from build123d import *

# Parameters (mm, degrees)
SKETCH1_R                = 7.9375
BOSS_EXTRUDE1_DEPTH      = 4.7625
H_0_266_DIAMETER_HOLE1_D = 6.7564


with BuildPart() as part:
    # Sketch1 → Boss-Extrude1 (new body)
    with BuildSketch(Plane.XY):
        with BuildLine():
            Line((-31.75, 0), (-50.274457233, 62.375531935))
            ThreePointArc((-50.274457233, 62.375531935), (-44.45, 76.989658396), (-28.881566614, 74.726723093))
            Line((-28.881566614, 74.726723093), (15.875, 27.49630657))
            Line((15.875, 27.49630657), (78.9111987, 12.409785423))
            Line((78.9111987, 12.409785423), (130.763159277, 0))
            Line((130.763159277, 0), (79.156023847, -12.351191158))
            Line((79.156023847, -12.351191158), (15.875, -27.49630657))
            Line((15.875, -27.49630657), (-28.881566614, -74.726723093))
            ThreePointArc((-28.881566614, -74.726723093), (-44.45, -76.989658396), (-50.274457233, -62.375531935))
            Line((-50.274457233, -62.375531935), (-31.75, 0))
        make_face()
        Circle(SKETCH1_R, mode=Mode.SUBTRACT)
        with BuildLine():
            Line((9.968214912, 24.497802386), (-25.925542767, 62.375531935))
            ThreePointArc((-25.925542767, 62.375531935), (-31.75, 54.99261314), (-41.056023847, 53.639944611))
            Line((-41.056023847, 53.639944611), (-26.199826659, 3.616173849))
            ThreePointArc((-26.199826659, 3.616173849), (-6.35, 10.998522628), (9.968214912, 24.497802386))
        make_face(mode=Mode.SUBTRACT)
        with BuildLine():
            Line((16.231611747, 20.881628537), (66.981566614, 8.735587325))
            ThreePointArc((66.981566614, 8.735587325), (63.5, 0), (66.981566614, -8.735587325))
            Line((66.981566614, -8.735587325), (16.231611747, -20.881628537))
            ThreePointArc((16.231611747, -20.881628537), (12.7, 0), (16.231611747, 20.881628537))
        make_face(mode=Mode.SUBTRACT)
        with BuildLine():
            Line((88.374457233, 3.615603833), (103.481579639, 0))
            Line((103.481579639, 0), (88.374457233, -3.615603833))
            ThreePointArc((88.374457233, -3.615603833), (88.9, 0), (88.374457233, 3.615603833))
        make_face(mode=Mode.SUBTRACT)
        with BuildLine():
            Line((9.968214912, -24.497802386), (-25.925542767, -62.375531935))
            ThreePointArc((-25.925542767, -62.375531935), (-31.75, -54.99261314), (-41.056023847, -53.639944611))
            Line((-41.056023847, -53.639944611), (-26.199826659, -3.616173849))
            ThreePointArc((-26.199826659, -3.616173849), (-6.35, -10.998522628), (9.968214912, -24.497802386))
        make_face(mode=Mode.SUBTRACT)
    extrude(amount=-BOSS_EXTRUDE1_DEPTH)

    # H (0.266) Diameter Hole1 (through all)
    with Locations(Plane.XY):
        with Locations((76.2, 0), (-38.1, 65.991135768), (-38.1, -65.991135768)):
            Hole(H_0_266_DIAMETER_HOLE1_D / 2)


solid = part.part
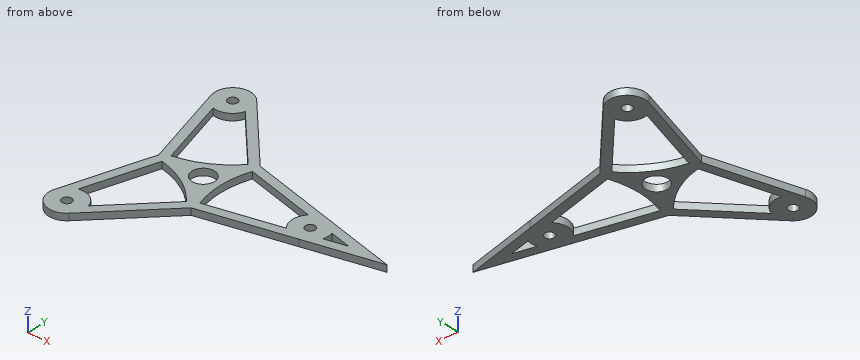
Here's how the part is built. I have some questions about the finished solid (model axes, mm). Give positions to 0.01 mm unless a question says otherwise; leave off trailing zeros. Loops run counter-clockwise (first coordinate to the right, second up) from the corner with the lowest first, then second, coordinate; pieces in that order, holes last. Notation, with made-up numbers: (68, 24) -> (101, 24) arc R24 ccw to (101, 52) -> close; hole circle Ø8 at (46.5, 2.5). An arc over 180 degrees is marked (long way). Answer as a JSON object with one key per item and string values. Group by question number.
Item 1: Imagine slicing it at A-A on x = -38.1. Write out the boundary of the cut face in (y, z), then the cut area to 3 significant figures.
Item 2: Will these pins go through, and if not, where does the flat tip stop? pin 1 (9 mm diameter, centred on x = -38.1, y = -65.99, fed in from +Z); pin 2 (1.5 mm diameter, centred on x = -3, z = -4, fed in from -Y).
Item 3: Imagine slicing it at C-C on y = -44. Write out the boundary of the cut face in (x, z).
Item 4: Imagine slicing it at D-D on z = -3.5. Give the number of separate pieces and of enclosed holes in the cut face, then the cut area to 3 significant figures.
Item 5: Imagine slicing it at B-B on x = 99.5. Write out the boundary of the cut face in (y, z).
Item 6: I need wall thicknesses on L1, parallel to Y at x = 9, z = -4.35; L2, parallel to Y at x = 0, z = -3.05; L3, parallel to Y at x = -2, z = -3.15. Which ranges of each line are inside material? Lowest first, please.
Answer list:
{
 "1": {"outline": "(-78.69, -4.76) -> (-69.37, -4.76) -> (-69.37, 0) -> (-78.69, 0) -> close; (-62.61, -4.76) -> (-53.29, -4.76) -> (-53.29, 0) -> (-62.61, 0) -> close; (-43.69, -4.76) -> (-21.38, -4.76) -> (-21.38, 0) -> (-43.69, 0) -> close; (21.38, -4.76) -> (43.69, -4.76) -> (43.69, 0) -> (21.38, 0) -> close; (53.29, -4.76) -> (62.61, -4.76) -> (62.61, 0) -> (53.29, 0) -> close; (69.37, -4.76) -> (78.69, -4.76) -> (78.69, 0) -> (69.37, 0) -> close", "area": "390 mm2"},
 "2": {"pin 1": "stops at z = 0", "pin 2": "stops at y = -48.21"},
 "3": {"outline": "(-44.82, -4.76) -> (-38.19, -4.76) -> (-38.19, 0) -> (-44.82, 0) -> close; (-8.51, -4.76) -> (0.24, -4.76) -> (0.24, 0) -> (-8.51, 0) -> close"},
 "4": {"separate pieces": "1", "enclosed holes": "8", "area": "4,830 mm2"},
 "5": {"outline": "(-7.48, -4.76) -> (-0.95, -4.76) -> (-0.95, 0) -> (-7.48, 0) -> close; (0.95, -4.76) -> (7.48, -4.76) -> (7.48, 0) -> (0.95, 0) -> close"},
 "6": {"L1": "y = -34.75 to -25.52, -23.4 to 23.4, 25.52 to 34.75", "L2": "y = -44.25 to -35.02, -15.19 to -7.94, 7.94 to 15.19, 35.02 to 44.25", "L3": "y = -46.36 to -37.13, -13.75 to -7.68, 7.68 to 13.75, 37.13 to 46.36"}
}
